```python
from build123d import *

# Parameters (mm, degrees)
HOLE1_D             = 9
HOLE2_D             = 9
SKETCH6_R           = 77.5
BOSS_EXTRUDE1_DEPTH = 5
CHAMFER1_SIZE       = 0.5


with BuildPart() as part:
    # Sketch1 → Revolve1 (revolve)
    with BuildSketch(Plane(origin=(0, 0, 0), x_dir=(1, 0, 0), z_dir=(0, 1, 0))):
        Polygon((105, 0), (0, 0), (0, -8), (104.5, -8), (105, -7.5), align=None)
    revolve(axis=Axis((0, 0, 0), (0, 0, 1)))

    # Hole1 (through all)
    with Locations(Plane.XY.offset(8)):
        with Locations((-47.5, -82.27241336), (-47.5, 82.27241336)):
            Hole(HOLE1_D / 2)

    # Hole2 (through all)
    with Locations(Plane(origin=(0, 0, 0), x_dir=(-1, 0, 0), z_dir=(0, 0, -1))):
        with Locations((-47.5, -82.27241336), (95, 0), (-47.5, 82.27241336), (-95, 0)):
            Hole(HOLE2_D / 2)

    # Sketch6 → Boss-Extrude1 (add)
    with BuildSketch(Plane.XY.offset(8)):
        Circle(SKETCH6_R)
    extrude(amount=BOSS_EXTRUDE1_DEPTH)

    # Chamfer1
    chamfer1_edges = [part.edges().sort_by_distance(p)[0] for p in [
        (-43, 82.27241336, 8),
        (-43, 82.27241336, 0),
        (-43, -82.27241336, 8),
        (-43, -82.27241336, 0),
        (90.5, 0, 0),
        (90.5, 0, 8),
        (43, 82.27241336, 0),
        (43, 82.27241336, 8),
        (-99.5, 0, 0),
        (-99.5, 0, 8),
        (43, -82.27241336, 0),
        (43, -82.27241336, 8),
        (-77.5, 0, 13),
        (-105, 0, 0),
    ]]
    chamfer(chamfer1_edges, length=CHAMFER1_SIZE)


solid = part.part
```
The listing builds one solid part. Answer for the finished solid, in the listing's coordinates (mm). Round coordinates to 2 decimals unless told otherwise and drop trailing zeros. Loops run counter-clockwise (first coordinate to the right, second up) from the corner with the lowest first, then second, coordinate; pieces in that order, holes last. Notation, with made-up numbers: (23.25, 84.25) -> (78.25, 84.25) arc R27 ccw to (78.25, 119.25) -> close; hole circle Ø6 at (-32, 23.5). An arc over 180 degrees is marked (long way). Use one line per item in the form item = value.
1. The part is cut by section B-B on x = -47.5. Give the number of separate pieces and of enclosed holes in the cut face, and give its area (3 significant figures).
Answer key:
separate_pieces = 3
enclosed_holes = 0
area = 1,960 mm²
2. Flat-ended cylindrical pins translate along their axes: pin 1 Ø10.5 at (x, y) = (-47.5, 82.27) entering from +Z; pin 2 Ø6 at (x, z) = (11, 9.5) entering from -Y; pin 3 Ø5 at (y, z) = (14, 11.5) entering from +X. Find the tip coordinate at first contact, or state that the pin passes through.
Answer key:
pin_1 = 8
pin_2 = -104.63
pin_3 = 76.64
3. Find the intervals of material crossed by probe 1 along Y at (x, z) = (-47.5, 4.75); probe 2 along Z at (x, y) = (-13.5, 81.5); probe 3 along X at (y, z) = (54, 3.75), in increasing order. Write a range as [from, to].
Answer key:
probe_1 = [-93.64, -86.77], [-77.77, 77.77], [86.77, 93.64]
probe_2 = [0, 8]
probe_3 = [-90.05, 90.05]
4. The part is cut by section A-A on z = 3.25. Determine the outline of the cut face in (x, y), and give its area (3 significant figures).
Answer key:
outline = circle Ø210 at (0, 0); hole circle Ø9 at (-95, 0); hole circle Ø9 at (-47.5, -82.27); hole circle Ø9 at (-47.5, 82.27); hole circle Ø9 at (47.5, -82.27); hole circle Ø9 at (47.5, 82.27); hole circle Ø9 at (95, 0)
area = 34,300 mm²
5. For a pull along Y with two mould halves and no side action, classify faces 1 (the cylindrical face through (90.504, 0.198, 4.049)), 2 (the cylindrical face through (100.15, 31.54, 3.95)), 3 (the flat face through (0, 78, 8)) as released by +Y, released by -Y, zero draft, split by the parting line, or undercut.
Answer key:
face_1 = undercut
face_2 = split by the parting line
face_3 = zero draft
